```python
from build123d import *

# Parameters (mm, degrees)
F0_R     = 6
F1_DEPTH = 15
F2_DEPTH = 45
F0_R_2   = 3
F3_DEPTH = 10


with BuildPart() as f1:
    # F0 (on Front) → F1 (new body)
    with BuildSketch(Plane.XZ):
        with BuildLine():
            Line((9.9873682983, 18.8420231841), (-40.0126317017, 18.8420231841))
            Line((-40.0126317017, 18.8420231841), (-40.0126317017, -0.3361211642))
            Line((-40.0126317017, -0.3361211642), (-38.5126317017, -0.3361211642))
            ThreePointArc((-38.5126317017, -0.3361211642), (-35.2908062948, 7.4420534289), (-27.5126317017, 10.6638788358))
            Line((-27.5126317017, 10.6638788358), (9.9873682983, 10.6638788358))
            Line((9.9873682983, 10.6638788358), (9.9873682983, 18.8420231841))
        make_face()
        with BuildLine():
            Line((59.9873682983, 18.8420231841), (9.9873682983, 18.8420231841))
            Line((9.9873682983, 18.8420231841), (9.9873682983, 10.6638788358))
            Line((9.9873682983, 10.6638788358), (47.4873682983, 10.6638788358))
            ThreePointArc((47.4873682983, 10.6638788358), (55.2655428913, 7.4420534289), (58.4873682983, -0.3361211642))
            Line((58.4873682983, -0.3361211642), (59.9873682983, -0.3361211642))
            Line((59.9873682983, -0.3361211642), (59.9873682983, 18.8420231841))
        make_face()
        with BuildLine():
            Line((-38.5126317017, -0.3361211642), (-40.0126317017, -0.3361211642))
            Line((-40.0126317017, -0.3361211642), (-40.0126317017, -21.1579768159))
            Line((-40.0126317017, -21.1579768159), (59.9873682983, -21.1579768159))
            Line((59.9873682983, -21.1579768159), (59.9873682983, -0.3361211642))
            Line((59.9873682983, -0.3361211642), (58.4873682983, -0.3361211642))
            ThreePointArc((58.4873682983, -0.3361211642), (55.2655428913, -8.1142957572), (47.4873682983, -11.3361211642))
            Line((47.4873682983, -11.3361211642), (-27.5126317017, -11.3361211642))
            ThreePointArc((-27.5126317017, -11.3361211642), (-35.2908062948, -8.1142957572), (-38.5126317017, -0.3361211642))
        make_face()
        with BuildLine():
            ThreePointArc((59.9873682983, -21.1579768159), (79.9873682983, -1.1579768159), (59.9873682983, 18.8420231841))
            Line((59.9873682983, 18.8420231841), (59.9873682983, -0.3361211642))
            Line((59.9873682983, -0.3361211642), (59.9873682983, -21.1579768159))
        make_face()
        with BuildLine():
            ThreePointArc((75.9873682983, -0.3361211642), (69.9873682983, -6.3361211642), (63.9873682983, -0.3361211642))
            ThreePointArc((63.9873682983, -0.3361211642), (69.9873682983, 5.6638788358), (75.9873682983, -0.3361211642))
        make_face(mode=Mode.SUBTRACT)
        with BuildLine():
            Line((-40.0126317017, -0.3361211642), (-40.0126317017, 18.8420231841))
            ThreePointArc((-40.0126317017, 18.8420231841), (-60.0126317017, -1.1579768159), (-40.0126317017, -21.1579768159))
            Line((-40.0126317017, -21.1579768159), (-40.0126317017, -0.3361211642))
        make_face()
        with Locations((-50.0126317017, -0.3361211642)):
            Circle(F0_R, mode=Mode.SUBTRACT)
    extrude(amount=F1_DEPTH)

    # F0 (on Front) → F2 (join)
    with BuildSketch(Plane.XZ):
        with BuildLine():
            Line((-27.5126317017, -7.8361211642), (-27.5126317017, -11.3361211642))
            Line((-27.5126317017, -11.3361211642), (47.4873682983, -11.3361211642))
            Line((47.4873682983, -11.3361211642), (47.4873682983, -7.8361211642))
            ThreePointArc((47.4873682983, -7.8361211642), (42.1840674394, -5.6394220231), (39.9873682983, -0.3361211642))
            Line((39.9873682983, -0.3361211642), (-20.0126317017, -0.3361211642))
            ThreePointArc((-20.0126317017, -0.3361211642), (-22.2093308428, -5.6394220231), (-27.5126317017, -7.8361211642))
        make_face()
        with BuildLine():
            Line((47.4873682983, 10.6638788358), (9.9873682983, 10.6638788358))
            Line((9.9873682983, 10.6638788358), (-27.5126317017, 10.6638788358))
            Line((-27.5126317017, 10.6638788358), (-27.5126317017, 7.1638788358))
            ThreePointArc((-27.5126317017, 7.1638788358), (-22.2093308428, 4.9671796947), (-20.0126317017, -0.3361211642))
            Line((-20.0126317017, -0.3361211642), (39.9873682983, -0.3361211642))
            ThreePointArc((39.9873682983, -0.3361211642), (42.1840674394, 4.9671796947), (47.4873682983, 7.1638788358))
            Line((47.4873682983, 7.1638788358), (47.4873682983, 10.6638788358))
        make_face()
        with BuildLine():
            ThreePointArc((-27.5126317017, 10.6638788358), (-35.2908062948, 7.4420534289), (-38.5126317017, -0.3361211642))
            Line((-38.5126317017, -0.3361211642), (-35.0126317017, -0.3361211642))
            ThreePointArc((-35.0126317017, -0.3361211642), (-32.8159325606, 4.9671796947), (-27.5126317017, 7.1638788358))
            Line((-27.5126317017, 7.1638788358), (-27.5126317017, 10.6638788358))
        make_face()
        with BuildLine():
            Line((-35.0126317017, -0.3361211642), (-38.5126317017, -0.3361211642))
            ThreePointArc((-38.5126317017, -0.3361211642), (-35.2908062948, -8.1142957572), (-27.5126317017, -11.3361211642))
            Line((-27.5126317017, -11.3361211642), (-27.5126317017, -7.8361211642))
            ThreePointArc((-27.5126317017, -7.8361211642), (-32.8159325606, -5.6394220231), (-35.0126317017, -0.3361211642))
        make_face()
        with BuildLine():
            ThreePointArc((47.4873682983, -11.3361211642), (55.2655428913, -8.1142957572), (58.4873682983, -0.3361211642))
            Line((58.4873682983, -0.3361211642), (54.9873682983, -0.3361211642))
            ThreePointArc((54.9873682983, -0.3361211642), (52.7906691572, -5.6394220231), (47.4873682983, -7.8361211642))
            Line((47.4873682983, -7.8361211642), (47.4873682983, -11.3361211642))
        make_face()
        with BuildLine():
            ThreePointArc((58.4873682983, -0.3361211642), (55.2655428913, 7.4420534289), (47.4873682983, 10.6638788358))
            Line((47.4873682983, 10.6638788358), (47.4873682983, 7.1638788358))
            ThreePointArc((47.4873682983, 7.1638788358), (52.7906691572, 4.9671796947), (54.9873682983, -0.3361211642))
            Line((54.9873682983, -0.3361211642), (58.4873682983, -0.3361211642))
        make_face()
    extrude(amount=F2_DEPTH)

    # F0 (on Front) → F3 (join)
    with BuildSketch(Plane.XZ):
        with BuildLine():
            ThreePointArc((75.9873682983, -0.3361211642), (69.9873682983, 5.6638788358), (63.9873682983, -0.3361211642))
            ThreePointArc((63.9873682983, -0.3361211642), (69.9873682983, -6.3361211642), (75.9873682983, -0.3361211642))
        make_face()
        with BuildLine():
            ThreePointArc((72.9873682983, -0.3361211642), (69.9873682983, -3.3361211642), (66.9873682983, -0.3361211642))
            ThreePointArc((66.9873682983, -0.3361211642), (69.9873682983, 2.6638788358), (72.9873682983, -0.3361211642))
        make_face(mode=Mode.SUBTRACT)
        with Locations((-50.0126317017, -0.3361211642)):
            Circle(F0_R)
        with Locations((-50.0126317017, -0.3361211642)):
            Circle(F0_R_2, mode=Mode.SUBTRACT)
    extrude(amount=F3_DEPTH)


solid = f1.part
```
Work out the finished part from the listing and answer in its coordinate system (mm). A direction names the side the tool comes from. Round coordinates to 2 decimals unless told otherwise and drop trailing zeros. Loops run counter-clockwise (first coordinate to the right, second up) from the corner with the lowest first, then second, coordinate; pieces in that order, holes last.
(1) Each of these flat-tipped pins is pushed along its axis until it touches: P1, Ø9, axis at x = -8, y = -30, coming from the -Z side; P2, Ø3.5, axis at x = -51.5, z = 2, coming from the -Y side; P3, Ø5, axis at y = -9, z = 11, coming from the -X side; P4, Ø9, axis at x = 47.49, z = -0.34, coming from the -Y side. Where does it stop, or does it pass through?
Computed values:
P1: stops at z = -11.34
P2: stops at y = -10
P3: stops at x = -57.53
P4: passes through
(2) For faces 1 (the cylindrical face through (-44.3, -12.5, 1.5)), 2 (the flat face through (11, -30, 10.664)), 3 (the flat face through (9, -30, -11.336)), determine the directions among +Z, -Z, +X, -X, +Y, -Y from which every point of the face is accessible in a straight line to the end or side of a thin tool.
Computed values:
face 1: -Y
face 2: +Z, +X, -X, -Y
face 3: -Z, +X, -X, -Y
(3) The part is cut by section B-B, the plane x = 49. Give the vertices of the cut face in (y, z).
Computed values:
outline: (-45, -11.23) - (-15, -11.23) - (-15, -21.16) - (0, -21.16) - (0, -7.68) - (-45, -7.68) - close; (-45, 7.01) - (0, 7.01) - (0, 18.84) - (-15, 18.84) - (-15, 10.56) - (-45, 10.56) - close
(4) The part is cut by section C-C, the plane y = -8. Give the vertices of the cut face in (x, z), and give its area (3 significant figures).
Computed values:
outline: (-40.01, -21.16) - (59.99, -21.16) arc R20 ccw to (59.99, 18.84) - (-40.01, 18.84) arc R20 ccw to start; hole circle Ø6 at (-50.01, -0.34); hole circle Ø15 at (-27.51, -0.34); hole circle Ø15 at (47.49, -0.34); hole circle Ø6 at (69.99, -0.34)
area: 4,850 mm2
(5) The part is cut by section A-A, the plane y = -25. Give the vertices of the cut face in (x, z), and give its area (3 significant figures).
Computed values:
outline: (-27.51, -11.34) - (47.49, -11.34) arc R11 ccw to (47.49, 10.66) - (-27.51, 10.66) arc R11 ccw to start; hole circle Ø15 at (-27.51, -0.34); hole circle Ø15 at (47.49, -0.34)
area: 1,680 mm2
(6) Find the intervals of material crossed by L1, parallel to X at y = -34.5, z = -1; L2, parallel to X at y = -5.5, z = -1; L3, parallel to X at y = -6, z = -4, in increasing order.
Computed values:
L1: x = -38.49 to -34.98, -20.04 to 40.02, 54.96 to 58.47
L2: x = -60.01 to -52.94, -47.09 to -34.98, -20.04 to 40.02, 54.96 to 67.06, 72.91 to 79.99
L3: x = -59.81 to -34.06, -20.97 to 40.94, 54.03 to 79.78
(7) The part is cut by section D-D, the plane x = 30.5. Give the vertices of the cut face in (y, z).
Computed values:
outline: (-45, -11.34) - (-15, -11.34) - (-15, -21.16) - (0, -21.16) - (0, 18.84) - (-15, 18.84) - (-15, 10.66) - (-45, 10.66) - close
(8) The mould has two halves that part along X. Classify faces 4 (the cylindrical face through (79.983, -7.395, -1.598)), 5 (the cylindrical face through (64.264, -12.465, 1.466)), 6 (the flat face through (9, -7, -21.158)): pulls with the +X half, pulls with the -X half, needs draft (parallel to the pull), parting line crosses it, or undercut.
Computed values:
face 4: pulls with the +X half
face 5: undercut
face 6: needs draft
